Can you work these out from the model? Positions are in its coordinate system, mm. A direction names the side the tool comes from. Coordinates: 2 decimals unless noted, no trailing zeros. Order: outer loops, then holes, each group sorted by start corner. A loop starts at its lowest first (then second) coordinate and runs counter-clockwise, first axis right, second up. Notation, with made-up numbers: (49.25, 34.5) -> (70.25, 34.5) arc R18 cw to (70.25, 58.5) -> close; hole circle Ø2 at (4, 86). An arc over 180 degrees is marked (long way). Return JSON: item names as keys, results as strings. Group by question number.
1) If we section it at D-D, the plane y = 3.75: Please give me the cut outline in (x, z), then the cut area to 3 significant figures.
2) If we section it at A-A, the plane x = 0: State how many separate pieces and enclosed holes the cut face has, then the cut area to 3 significant figures.
3) If we section it at B-B, the plane y = 7.5: Please give me the cut outline in (x, z), then the cut area to 3 significant figures.
4) Thinking about a two-plate mould opening in Z: for faces 6 (the cylindrical face through (0.07, -2.235, -1.42)), 7 (the conical face through (-1.16, 3.11, -8.87)), 8 (the flat face through (0, 1, -3.114)), 9 (the flat face through (-7, 0, -2)), which applies, +Z half, -Z half, draft (parallel to the pull), parting line (faces both ways), or undercut?
5) For pin 1 (10 mm diameter, centred on x = 3, z = 2.5, fed in from -Y); pin 2 (5 mm diameter, centred on x = 3, y = 0, fed in from +Z); pin 3 (1.2 mm diameter, centred on x = 7, z = -1, fed in from -Y), each with a flat end and sliding along its axis, tell me the tip position at first contact or that it passes through.
6) If I drill on probe 1 along Z at (x, y) = (2.75, -2.5); probe 2 along Y at (x, z) = (-7.5, -4.25); probe 3 along Z at (x, y) = (-3.75, -1.25), over which ranges is the centre line in solid material (lowest first)? Write a range as from..to.
7) For faces 1 (the flat face through (-0.1, -0.5, 1.886)), 2 (the flat face through (-4, 1, -5)), 3 (the flat face through (7, 0, -2)), 4 (the flat face through (-5, -3, -4)), 5 (the flat face through (0, 9.117, 0)), which set-ups out of +Z, -Z, +X, -X, +Y, -Y let a thin tool reach every point of the face, with its end or its side?
from build123d import *

# Parameters (mm, degrees)
SKETCH1_R                     = 9
BOSS_EXTRUDE1_DEPTH           = 19
BOSS_EXTRUDE1_TAPER           = 1
BOSS_EXTRUDE1_OTHER_WAY_DEPTH = 6
BOSS_EXTRUDE1_OTHER_WAY_TAPER = -1
CUT_EXTRUDE1_DEPTH            = 23.951954839
CUT_EXTRUDE1_DEPTH_BACK       = 23.951954839
SKETCH4_W                     = 6.502745185
SKETCH4_H                     = 6
CUT_EXTRUDE2_DEPTH            = 24.763281499
SKETCH5_R                     = 1.5
CUT_EXTRUDE3_DEPTH            = 26.296168166
FILLET1_SIZE                  = 5
CUT_EXTRUDE4_DEPTH            = 23.910611578
CUT_EXTRUDE4_DEPTH_BACK       = 23.910611578
SKETCH6_W                     = 24.694280634
SKETCH6_H                     = 10.883453579
CUT_EXTRUDE5_DEPTH            = 20.809242737


with BuildPart() as part:
    # Sketch1 → Boss-Extrude1 (new body)
    with BuildSketch(Plane(origin=(0, 0, 0), x_dir=(1, 0, 0), z_dir=(0, 1, 0))):
        Circle(SKETCH1_R)
    extrude(amount=BOSS_EXTRUDE1_DEPTH, taper=BOSS_EXTRUDE1_TAPER)

    # Sketch1 → Boss-Extrude1 other way (add)
    with BuildSketch(Plane(origin=(0, 0, 0), x_dir=(1, 0, 0), z_dir=(0, 1, 0))):
        Circle(SKETCH1_R)
    extrude(amount=-BOSS_EXTRUDE1_OTHER_WAY_DEPTH, taper=BOSS_EXTRUDE1_OTHER_WAY_TAPER)

    # Sketch3 → Cut-Extrude1 (cut, two sides: drawn at the far end of the back side and taken through both)
    with BuildSketch(Plane(origin=(0, 0, 0), x_dir=(0, 0, -1), z_dir=(1, 0, 0)).offset(-CUT_EXTRUDE1_DEPTH_BACK)):
        Polygon((-1.886057768, -6), (-1.886057768, 0), (-9.929766736, 8.043708969), (-9.929766736, -6), align=None)
    extrude(amount=CUT_EXTRUDE1_DEPTH + CUT_EXTRUDE1_DEPTH_BACK, mode=Mode.SUBTRACT)

    # Sketch4 → Cut-Extrude2 (cut, through all)
    with BuildSketch(Plane.XY.offset(1.886057768)):
        with Locations((-8.251372593, -3)):
            Rectangle(SKETCH4_W, SKETCH4_H)
        with Locations((8.251372593, -3)):
            Rectangle(SKETCH4_W, SKETCH4_H)
    extrude(amount=-CUT_EXTRUDE2_DEPTH, mode=Mode.SUBTRACT)

    # Sketch5 → Cut-Extrude3 (cut, through all)
    with BuildSketch(Plane(origin=(5, 0, 0), x_dir=(0, 0, -1), z_dir=(1, 0, 0))):
        with Locations((0.613942232, -3.5)):
            Circle(SKETCH5_R)
    extrude(amount=-CUT_EXTRUDE3_DEPTH, mode=Mode.SUBTRACT)

    # Fillet1
    # a fillet whose section is not a circle: 5 mm, written as the material it takes off along each edge
    with BuildSketch(Plane(origin=(17.5, -6, 1.886057768), x_dir=(0, 0, -1), z_dir=(-1, 0, 0))) as fillet1_piece_1:
        with BuildLine():
            Bezier((FILLET1_SIZE, 0), (0, 0), (0, -FILLET1_SIZE), weights=[1, 1.5, 1])
            Line((0, -FILLET1_SIZE), (0, 0))
            Line((0, 0), (FILLET1_SIZE, 0))
        make_face()
    extrude(amount=35, mode=Mode.SUBTRACT)

    # Fillet2
    # a fillet whose section is not a circle: 10, 5 mm, written as the material it takes off along each edge
    with BuildSketch(Plane(origin=(0, 19, 0), x_dir=(1, 0, 0), z_dir=(0, 0, -1))) as fillet2_piece_1:
        with BuildLine():
            Bezier((8.841381251, 9.912737968), (8.668353766, 0), (3.842142775, 0), weights=[1, 0.818181818, 1])
            Line((3.842142775, 0), (8.668353766, 0))
            Line((8.668353766, 0), (8.841381251, 9.912737968))
        make_face()
    revolve(axis=Axis((0, 19, 0), (0, -1, 0)), mode=Mode.SUBTRACT)

    # Sketch6 → Cut-Extrude4 (cut, two sides: drawn at the far end of the back side and taken through both)
    with BuildSketch(Plane(origin=(0, 0, 0), x_dir=(0, 0, -1), z_dir=(1, 0, 0)).offset(-CUT_EXTRUDE4_DEPTH_BACK)):
        with Locations((1.854254765, 14.558273211)):
            Rectangle(SKETCH6_W, SKETCH6_H)
    extrude(amount=CUT_EXTRUDE4_DEPTH + CUT_EXTRUDE4_DEPTH_BACK, mode=Mode.SUBTRACT)

    # Sketch7 → Cut-Extrude5 (cut, through all)
    with BuildSketch(Plane.XZ.offset(6)):
        with BuildLine():
            Line((4, -3.113942232), (4, -5.871728358))
            ThreePointArc((4, -5.871728358), (0, -7.10473039), (-4, -5.871728358))
            Line((-4, -5.871728358), (-4, -3.113942232))
            Line((-4, -3.113942232), (4, -3.113942232))
        make_face()
    extrude(amount=-CUT_EXTRUDE5_DEPTH, mode=Mode.SUBTRACT)


solid = part.part
Result sheet:
{
 "1": {"outline": "(-6.93, 5.64) arc R8.93 ccw (long way) to (6.93, 5.64) -> close; hole (-4, -5.87) arc R7.1 ccw to (4, -5.87) -> (4, -3.11) -> (-4, -3.11) -> close", "area": "190 mm2"},
 "2": {"separate pieces": "2", "enclosed holes": "1", "area": "133 mm2"},
 "3": {"outline": "circle Ø17.74 at (0, 0); hole (-4, -5.87) arc R7.1 ccw to (4, -5.87) -> (4, -3.11) -> (-4, -3.11) -> close", "area": "218 mm2"},
 "4": {"face 6": "undercut", "face 7": "parting line", "face 8": "undercut", "face 9": "draft"},
 "5": {"pin 1": "stops at y = -5.99", "pin 2": "stops at z = 4.39", "pin 3": "stops at y = 0"},
 "6": {"probe 1": "z = -8.62..-6.55, -3.11..-1.73, 0.5..1.82", "probe 2": "y = 0..9.12", "probe 3": "z = -8.21..-6.03, -3.11..1.88"},
 "7": {"face 1": "+Z, +X, -X, -Y", "face 2": "+Y, -Y", "face 3": "+Z, -Z, +X, -Y", "face 4": "+Z, -Z, -X, -Y", "face 5": "+Z, -Z, +X, -X, +Y"}
}
